```python
from build123d import *

# Parameters (mm, degrees)
CROQUIS1_W              = 40
CROQUIS1_H              = 40
CROQUIS1_R              = 1.35
SALIENTE_EXTRUIR1_DEPTH = 10
CROQUIS2_R              = 10
CROQUIS2_R_2            = 1.9
SALIENTE_EXTRUIR2_DEPTH = 8


with BuildPart() as part:
    # Croquis1 → Saliente-Extruir1 (new body)
    with BuildSketch(Plane(origin=(0, 0, 0), x_dir=(1, 0, 0), z_dir=(0, 1, 0))):
        Rectangle(CROQUIS1_W, CROQUIS1_H)
        with Locations(Location((-10, 10, 0), (0, 0, 270))):
            Circle(CROQUIS1_R, mode=Mode.SUBTRACT)
        with Locations(Location((10, 10, 0), (0, 0, 90))):
            Circle(CROQUIS1_R, mode=Mode.SUBTRACT)
        with Locations(Location((10, -10, 0), (0, 0, 270))):
            Circle(CROQUIS1_R, mode=Mode.SUBTRACT)
        with Locations(Location((-10, -10, 0), (0, 0, 90))):
            Circle(CROQUIS1_R, mode=Mode.SUBTRACT)
    extrude(amount=SALIENTE_EXTRUIR1_DEPTH)

    # Croquis2 → Saliente-Extruir2 (add)
    with BuildSketch(Plane(origin=(0, 0, -20), x_dir=(-1, 0, 0), z_dir=(0, 0, -1))):
        Circle(CROQUIS2_R)
        with Locations((0, -6)):
            Circle(CROQUIS2_R_2, mode=Mode.SUBTRACT)
    extrude(amount=-SALIENTE_EXTRUIR2_DEPTH)


solid = part.part
```
Work out the finished part from the listing and answer in its coordinate system (mm). A direction names the side the tool comes from. Round coordinates to 2 decimals unless told otherwise and drop trailing zeros. Write each loop counter-clockwise with the first axis right and the second up, starting at its lowest first coordinate (ties: lowest second). Pieces come first, ordered by that corner, then holes.
1) A cutting plane is placed at A-A on y = -6. Determine the outline of the cut face in (x, z).
2) Consider probe 1 along X at (y, z) = (4.5, -10); probe 2 along Y at (x, z) = (0, -17); probe 3 along Z at (x, y) = (-9, 8.75). Determine where each line is inside the solid, lowest interval first.
3) Flat-ended cylindrical pins translate along their axes: P1, Ø3.5, axis at x = 10, z = -10, coming from the +Y side; P2, Ø12, axis at x = -0.5, z = -5, coming from the -Y side; P3, Ø4, axis at y = -6.5, z = -10.5, coming from the +X side; P4, Ø8, axis at x = 2.5, y = -7, coming from the +Z side. Find the tip coordinate at first contact, or state that the pin passes through.
4) A cutting plane is placed at B-B on z = 10. Determine the outline of the cut face in (x, y), and give its area (3 significant figures).
5) A cutting plane is placed at D-D on x = 6. Determine the outline of the cut face in (y, z).
6) Which of the six approach directions +Z, -Z, +X, -X, +Y, -Y give full straight-line access (tool end or side, diameter ignored) to faces 1 (the face through (0, 2, -20)), 2 (the face through (0.1, -3.8, -12))?
7) A cutting plane is placed at C-C on x = 0. Determine the outline of the cut face in (y, z), and give its area (3 significant figures).
8) Determine the mould class of faces 3 (the face through (-11.339, 4.93, 10.176)), 4 (the face through (0, 10, 0)), 5 (the face through (0, 5, 20)) for opening direction Z: pulls with the +Z half, pulls with the -Z half, needs draft (parallel to the pull), parting line crosses it, or undercut.
Entries:
1. outline: (-8, -20) - (-1.9, -20) - (-1.9, -12) - (-8, -12) - close; (1.9, -20) - (8, -20) - (8, -12) - (1.9, -12) - close
2. probe 1: x = -20 to -11.35, -8.65 to 8.65, 11.35 to 20
2. probe 2: y = -10 to -7.9, -4.1 to 10
2. probe 3: z = -20 to -10.91, -9.09 to 9.09, 10.91 to 20
3. P1: stops at y = 10
3. P2: stops at y = 0
3. P3: stops at x = 8.56
3. P4: stops at z = -12
4. outline: (-20, 0) - (-11.35, 0) - (-11.35, 10) - (-20, 10) - close; (-8.65, 0) - (8.65, 0) - (8.65, 10) - (-8.65, 10) - close; (11.35, 0) - (20, 0) - (20, 10) - (11.35, 10) - close
4. area: 346 mm2
5. outline: (-8, -20) - (10, -20) - (10, 20) - (0, 20) - (0, -12) - (-8, -12) - close
6. face 1: -Z, +X, -X, +Y, -Y
6. face 2: +Z, +X, -X, -Y
7. outline: (-10, -20) - (-7.9, -20) - (-7.9, -12) - (-10, -12) - close; (-4.1, -20) - (10, -20) - (10, 20) - (0, 20) - (0, -12) - (-4.1, -12) - close
7. area: 450 mm2
8. face 3: undercut
8. face 4: needs draft
8. face 5: pulls with the +Z half
